Part model, mm, in its own coordinate system. Face numbers are marked on the shaded views. A direction names the side the tool comes from. Give positions to 0.01 mm unless a question says otherwise; leave off trailing zeros. Order: outer loops, then holes, each group sorted by start corner. A loop starts at its lowest first (then second) coordinate and runs counter-clockwise, first axis right, second up. Notation, with made-up numbers: (-28, -16) - (-24, -16) arc R8 cw to (-24, -5) - close; hole circle Ø10 at (75.5, 16). An arc over 180 degrees is marked (long way). One line per item, written item: value.
```python
from build123d import *

# Parameters (mm, degrees)
F0_W     = 304.8
F0_H     = 203.2
F1_DEPTH = 254
F2_W     = 254
F2_H     = 203.2
F3_DEPTH = 6.35
F7_DEPTH = 95.491579


with BuildPart() as f1:
    # F0 (on Front) → F1 (new body)
    with BuildSketch(Plane.XZ):
        with Locations((457.2, 304.8)):
            Rectangle(F0_W, F0_H)
        Polygon((609.6, 203.2), (914.4, 203.2), (914.4, 609.6), (609.6, 609.6), (609.6, 406.4), align=None)
        Polygon((0, 203.2), (0, 0), (914.4, 0), (914.4, 203.2), (609.6, 203.2), (304.8, 203.2), align=None)
    extrude(amount=F1_DEPTH)

    # F2 (on face) → F3 (cut)
    with BuildSketch(Plane.XY.offset(203.2)):
        with Locations((152.4, -127)):
            Rectangle(F2_W, F2_H)
    extrude(amount=-F3_DEPTH, mode=Mode.SUBTRACT)

    # F6 (on offset) → F7 (join)
    with BuildSketch(Plane.XZ.offset(127)):
        with BuildLine():
            ThreePointArc((273.291586, 208.28), (152.400003, 212.119769), (31.50842, 208.28))
            ThreePointArc((31.50842, 208.28), (27.022893, 203.329925), (25.4, 196.85))
            Line((25.4, 196.85), (279.4, 196.85))
            ThreePointArc((279.4, 196.85), (277.777109, 203.329923), (273.291586, 208.28))
        make_face()
    extrude(amount=F7_DEPTH)


solid = f1.part
```
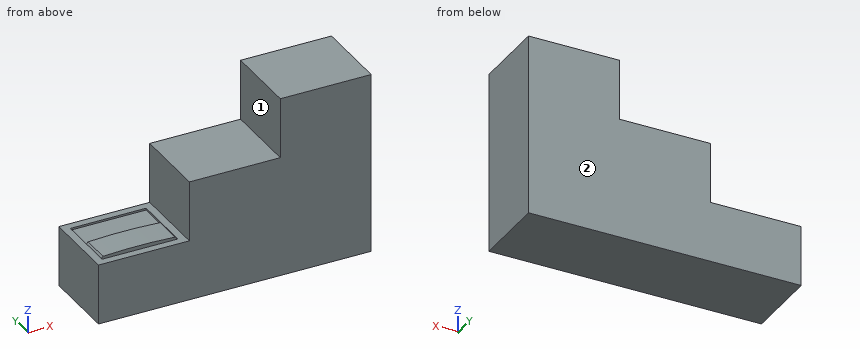
1) Slice it at D-D on y = -61.5. Write the cut outline in (x, z), then the cut area to 3 significant figures.
Answer:
outline: (0, 0) - (914.4, 0) - (914.4, 609.6) - (609.6, 609.6) - (609.6, 406.4) - (304.8, 406.4) - (304.8, 203.2) - (279.4, 203.2) - (279.4, 196.85) - (25.4, 196.85) - (25.4, 203.2) - (0, 203.2) - close
area: 370,000 mm2
2) Slice it at B-B on x = 183.5. Write the cut outline in (y, z).
Answer:
outline: (-254, 0) - (0, 0) - (0, 203.2) - (-25.4, 203.2) - (-25.4, 196.85) - (-127, 196.85) - (-127, 211.87) - (-222.49, 211.87) - (-222.49, 196.85) - (-228.6, 196.85) - (-228.6, 203.2) - (-254, 203.2) - close
3) Drop flat-ended pins along their axis: P1, Ø2, axis at y = -108.5, z = 434, coming from the -X side; P2, Ø1.5, axis at x = 276, y = -223, coming from the +Z side; P3, Ø6, axis at x = 362.5, y = -48, coming from the +Z side. Give the stop position or say it passes through.
Answer:
P1: stops at x = 609.6
P2: stops at z = 206.5
P3: stops at z = 406.4
4) Wall check: line 1 along Z through (x, y) = (365.5, -23); line 2 along Z through (x, y) = (304, -20); line 3 along X through (y, z) = (-69, 450.5). Give the ranges that are in metal, low to high. Write a range as [from, to].
Answer:
line 1: z = [0, 406.4]
line 2: z = [0, 203.2]
line 3: x = [609.6, 914.4]
5) Which spindle directions (+Z, -Z, +X, -X, +Y, -Y) get a long thin tool onto all of the face, cutting with end or side? Do the marked faces 1 and 2. Say none if no direction does.
Answer:
face 1: +Z, -X, +Y, -Y
face 2: +Z, -Z, +X, -X, +Y
6) Slice it at A-A on y = -188. Write the cut outline in (x, z).
Answer:
outline: (0, 0) - (914.4, 0) - (914.4, 609.6) - (609.6, 609.6) - (609.6, 406.4) - (304.8, 406.4) - (304.8, 203.2) - (279.4, 203.2) - (279.4, 196.85) arc R13.75 ccw to (273.29, 208.28) arc R1905 ccw to (31.51, 208.28) arc R13.75 ccw to (25.4, 196.85) - (25.4, 203.2) - (0, 203.2) - close
7) Slice it at C-C on z = 564. Write the cut outline in (x, y), then the cut area to 3 significant figures.
Answer:
outline: (609.6, -254) - (914.4, -254) - (914.4, 0) - (609.6, 0) - close
area: 77,400 mm2
